Can you work these out from the model? Positions are in its coordinate system, mm. A direction names the side the tool comes from. Round coordinates to 2 decimals unless told otherwise and drop trailing zeros. Loops run counter-clockwise (first coordinate to the right, second up) from the corner with the lowest first, then second, coordinate; pieces in that order, holes last. Notation, with made-up numbers: (87.5, 4) -> (102.5, 4) arc R18 cw to (102.5, 37) -> close; hole circle Ø4 at (-30, -31). An arc over 180 degrees is marked (long way). Use a Markdown table: item, result.
Autodesk Inventor part; units mm, degrees
ref_plane "YZ Plane" through (0, 0, 0) normal (1, 0, 0) x (0, 1, 0)
ref_plane "XZ Plane" through (0, 0, 0) normal (0, 1, 0) x (-1, 0, 0)
ref_plane "XY Plane" through (0, 0, 0) normal (0, 0, 1) x (1, 0, 0)
sketch "Эскиз3" plane through (0, 0, 0) normal (0, 1, 0) x (-1, 0, 0)
  arc A0 (1.791, 3.5766) -> (0.2774, -3.9904) centre (0, 0) ccw
  arc A1 (14, -20) -> (1.791, 3.5766) centre (-14.2382, -19.6735) ccw
  arc A2 (8, -20) -> (0.2774, -3.9904) centre (-13.4368, -20.4731) ccw
  line L0 (8, -20) -> (14, -20)
  line L1 (0, 0) -> (13.752, 0)
  dimension "d12" = 8
  dimension "d27" = 8
  dimension "d29" = 20
  dimension "d30" = 6
extrude "Выдавливание5" add sketch "Эскиз3" along normal blind 3
sketch "Эскиз5" plane through (0, 3, 0) normal (0, 1, 0) x (1, 0, 0)
  circle A0 centre (0, 0) radius 2
  dimension "d24" = 4
extrude "Выдавливание6" cut sketch "Эскиз5" against normal blind 10
mirror "Зеркальное отражение1" about plane through (-8, 0, -20) normal (0, 0, -1) of "Выдавливание5", "Выдавливание6"
properties part number "000.703 - Тяга" material "Пластик АБС"
1. I want a section at A-A (y = 1.95). Please give me the cut outline in (x, z).
Answer sheet:
| item | result |
|---|---|
| outline | (-14, -20) arc R28.24 ccw to (-1.79, -43.58) arc R4 ccw (long way) to (-0.28, -36.01) arc R21.44 cw to (-8, -20) arc R21.44 cw to (-0.28, -3.99) arc R4 ccw (long way) to (-1.79, 3.58) arc R28.24 ccw to start; hole circle Ø4 at (0, -40); hole circle Ø4 at (0, 0) |
2. I need wall thicknesses on line 1 (Z direction, x = 0, y = 1.7); line 2 (Z direction, x = -1.5, y = 1.15); line 3 (X direction, y = 1.1, z = -40). Which ranges of each line are inside material? Lowest first, please.
Answer sheet:
| item | result |
|---|---|
| line 1 | z = -44 to -42, -38 to -36, -4 to -2, 2 to 4 |
| line 2 | z = -43.71 to -41.32, -38.68 to -34.91, -5.09 to -1.32, 1.32 to 3.71 |
| line 3 | x = -6.02 to -2, 2 to 4 |
3. I want a section at B-B (x = 0.5). Please give me the cut outline in (y, z).
Answer sheet:
| item | result |
|---|---|
| outline | (0, -43.97) -> (3, -43.97) -> (3, -41.94) -> (0, -41.94) -> close; (0, -38.06) -> (3, -38.06) -> (3, -36.03) -> (0, -36.03) -> close; (0, -3.97) -> (3, -3.97) -> (3, -1.94) -> (0, -1.94) -> close; (0, 1.94) -> (3, 1.94) -> (3, 3.97) -> (0, 3.97) -> close |
4. I want a section at D-D (x = -6.25). Please give me the cut outline in (y, z).
Answer sheet:
| item | result |
|---|---|
| outline | (0, -39.76) -> (3, -39.76) -> (3, -28.02) -> (0, -28.02) -> close; (0, -11.98) -> (3, -11.98) -> (3, -0.24) -> (0, -0.24) -> close |
5. Which directions (+Z, -Z, +X, -X, +Y, -Y) give clear straight access to the entire face, cutting with the end or side of a thin tool? Please do faces 3 (the flat face through (-9, 0, -20)), 4 (the cylindrical face through (-5.8, 1.5, -11)).
Answer sheet:
| item | result |
|---|---|
| face 3 | +Z, -Z, +X, -X, -Y |
| face 4 | +X, +Y, -Y |
6. I want a section at C-C (z = -40). Please give me the cut outline in (x, y), plus the area to 3 significant figures.
Answer sheet:
| item | result |
|---|---|
| outline | (-6.02, 0) -> (-2, 0) -> (-2, 3) -> (-6.02, 3) -> close; (2, 0) -> (4, 0) -> (4, 3) -> (2, 3) -> close |
| area | 18.1 mm² |
7. If we mould it in two halves opening along Z, with no side actions, what happens to faces 1 (the cylindrical face through (0, 2, 2)), 2 (the flat face through (-9, 3, -20))? For each: +Z half, -Z half, draft (parallel to the pull), parting line (faces both ways), or undercut.
Answer sheet:
| item | result |
|---|---|
| face 1 | undercut |
| face 2 | draft |
8. Will these pins go through, and if not, where does the flat tip stop? pin 1 Ø3 at (x, z) = (0, -40) entering from -Y (3 decimals); pin 2 Ø1 at (x, y) = (-7, 2.5) entering from -Z.
Answer sheet:
| item | result |
|---|---|
| pin 1 | passes through |
| pin 2 | stops at z = -39.49 |
